Source: three-view drawing plus pictorial views. Frame: mm from the lowest corner of the part. Coordinates: 2 decimals unless noted, no trailing zeros. Order: outer loops, then holes, each group sorted by start corner. A loop starts at its lowest first (then second) coordinate and runs counter-clockwise, first axis right, second up. Notation, with made-up numbers: (32, 65.25) -> (68, 65.25) arc R14 ccw to (68, 83.25) -> close; hole circle Ø7 at (32, 52). An arc over 180 degrees is marked (long way). Use CSV: the item, a comma, the result in double quotes. Start each with the question number.
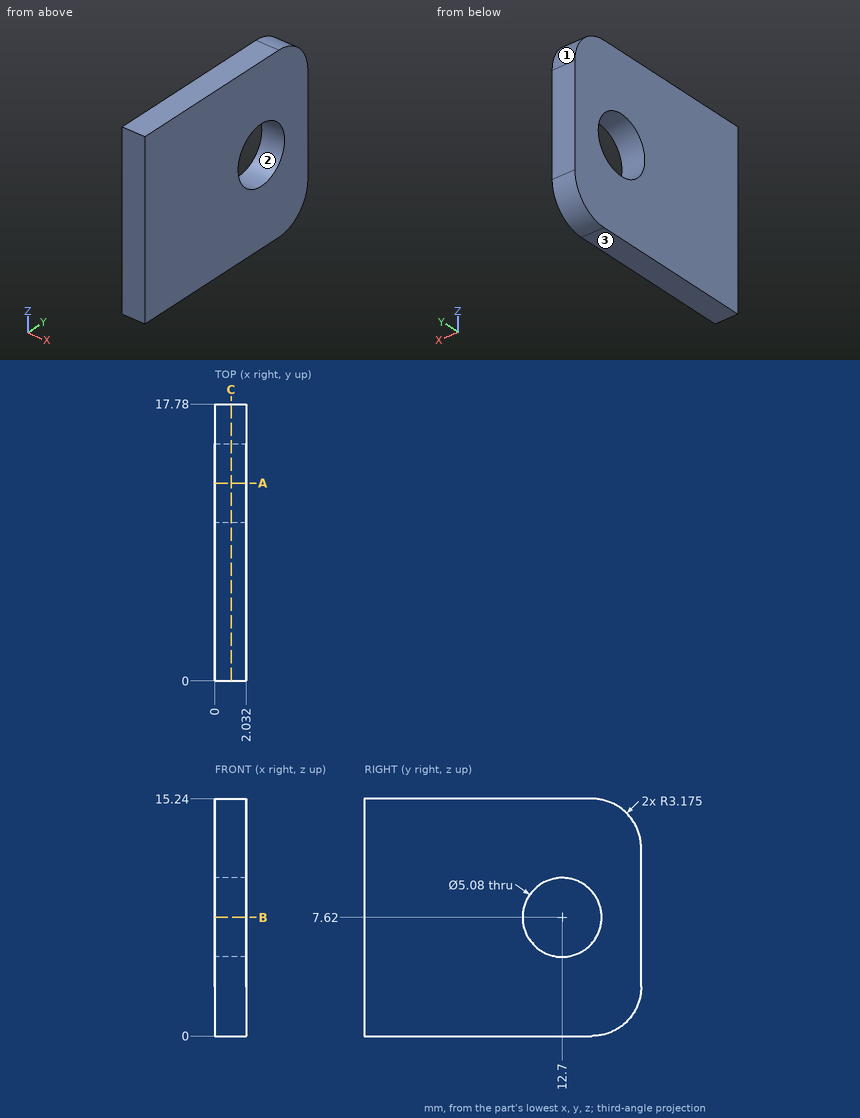
1. Pull-direction query (Y, two-part tool) for the marked faces 1, 2 and 3; classes: released by +Y, released by -Y, zero draft, split by the parting line, or undercut.
2. Material intervals for line 1 along Z through (x, y) = (0.55, 12.7); line 2 along Y through (x, z) = (1.3, 9.5); line 3 along Y through (x, z) = (0.3, 5.5), sorted ascending.
3. Section A-A on y = 12.7. Return loops of the section in (x, z).
4. Section B-B on z = 7.62. Return loops of the section in (x, y).
5. Section C-C on x = 1.05. Return loops of the section in (y, z) (3 decimals), then the cut area to 3 significant figures.
6. Contact query for flat-ended pins moving along their axis: P1, Ø3, axis at y = 12.7, z = 7.62, coming from the -X side; P2, Ø4, axis at y = 7, z = 11, coming from the -X side. Output: stop coordinate, or through.
Values follow:
1,face 1,"released by +Y"
1,face 2,"undercut"
1,face 3,"zero draft"
2,line 1,"z = 0 to 5.08, 10.16 to 15.24"
2,line 2,"y = 0 to 10.99, 14.41 to 17.78"
2,line 3,"y = 0 to 11.3, 14.1 to 17.78"
3,outline,"(0, 0) -> (2.03, 0) -> (2.03, 5.08) -> (0, 5.08) -> close; (0, 10.16) -> (2.03, 10.16) -> (2.03, 15.24) -> (0, 15.24) -> close"
4,outline,"(0, 0) -> (2.03, 0) -> (2.03, 10.16) -> (0, 10.16) -> close; (0, 15.24) -> (2.03, 15.24) -> (2.03, 17.78) -> (0, 17.78) -> close"
5,outline,"(0, 0) -> (14.605, 0) arc R3.175 ccw to (17.78, 3.175) -> (17.78, 12.065) arc R3.175 ccw to (14.605, 15.24) -> (0, 15.24) -> close; hole circle Ø5.08 at (12.7, 7.62)"
5,area,"246 mm2"
6,P1,"passes through"
6,P2,"stops at x = 0"
